Model file for the job. Use its own axes, mm. A direction names the side the tool comes from. Round coordinates to 2 decimals unless told otherwise and drop trailing zeros. Order: outer loops, then holes, each group sorted by start corner. A loop starts at its lowest first (then second) coordinate and runs counter-clockwise, first axis right, second up. Notation, with made-up numbers: (7, -31) - (66, -31) arc R18 ccw to (66, -23) - close; hole circle Ø2 at (-7, 54). An arc over 180 degrees is marked (long way). Put each result on its own line as item: value. Start each with the question number.
Item 1: Pin check, flat tip, straight feed: pin 1 Ø1 at (x, y) = (-16.5, 34) entering from +Z. Stop position of the tip, or through.
Item 2: Probe probe 1 along Y at (x, z) = (-40.5, 0.5); probe 2 along Y at (x, z) = (-11, 4); probe 3 along Y at (x, z) = (14, 2). List the from-to ranges inside material, lowest first.
Item 3: Which spindle directions (+Z, -Z, +X, -X, +Y, -Y) get a long thin tool onto all of the face, cutting with end or side? Do faces 1 (the face through (0, -32, 2)), 2 (the face through (2, -12.278, 2)). Say none if no direction does.
Item 4: Saw through at C-C on y = -10.5. List the corners of the cut face in (x, z), plus the area to 3 significant figures.
Item 5: Saw through at D-D on x = -43.5. List the corners of the cut face in (y, z).
Item 6: Mould opens along X. For faces 3 (the face through (1, -56.48, 2)), 4 (the face through (-38, -26.567, 2)) say: pulls with the +X half, pulls with the -X half, needs draft (parallel to the pull), parting line crosses it, or undercut.
Item 7: Saw through at A-A on x = 9. List the corners of the cut face in (y, z).
Item 8: Saw through at B-B on z = 2. List the corners of the cut face in (x, y), plus the area to 3 significant figures.
```python
from build123d import *

# Parameters (mm, degrees)
F1_DEPTH = 5
F2_DEPTH = 2


# Not quite as in the source:
# - a feature names something its author has since deleted; it is built from what else it names


with BuildPart() as f1:
    # F0 (on Top) → F1 (new body)
    with BuildSketch(Plane.XY):
        Polygon((-53.2781591106, 53.5204063327), (-53.2781591106, -56.4795936673), (-13.7344817631, -56.4795936673), (56.7218408894, -56.4795936673), (56.7218408894, 53.5204063327), align=None)
        Polygon((-49.0473898798, 29.4351325184), (-49.0473898798, 49.289637102), (52.4910716586, 49.289637102), (52.4910716586, 29.4351325184), (27.9224817305, -52.2488244365), (-13.7344817631, -52.2488244365), (-13.7344817631, -40.6398742527), (-26.4708319562, -40.6398742527), (-26.4708319562, -26.5670741801), (-49.0473898798, -26.5670741801), (-49.0473898798, 5.428542512), (-49.0473898798, 25.9305896417), (-26.4708319562, 25.9305896417), (13.9133328608, 25.9305896417), (13.9133328608, 5.428542512), (13.9133328608, -12.2777693511), (-9.5037125323, -12.2777693511), (-9.5037125323, 5.428542512), (-26.4708319562, 5.428542512), (-26.4708319562, -12.2777693511), (-13.7344817631, -12.2777693511), (-13.7344817631, -26.5670741801), (0, -26.5670741801), (0, -37.4845501322), (17.3598656954, -37.4845501322), (37.487713347, 29.4351325184), align=None, mode=Mode.SUBTRACT)
    extrude(amount=F1_DEPTH)

    # F0 (on Top) → F2 (join)
    with BuildSketch(Plane.XY):
        Polygon((-53.2781591106, 53.5204063327), (-53.2781591106, -56.4795936673), (-13.7344817631, -56.4795936673), (56.7218408894, -56.4795936673), (56.7218408894, 53.5204063327), align=None)
        Polygon((-49.0473898798, 29.4351325184), (-49.0473898798, 49.289637102), (52.4910716586, 49.289637102), (52.4910716586, 29.4351325184), (27.9224817305, -52.2488244365), (-13.7344817631, -52.2488244365), (-13.7344817631, -40.6398742527), (-26.4708319562, -40.6398742527), (-26.4708319562, -26.5670741801), (-49.0473898798, -26.5670741801), (-49.0473898798, 5.428542512), (-49.0473898798, 25.9305896417), (-26.4708319562, 25.9305896417), (13.9133328608, 25.9305896417), (13.9133328608, 5.428542512), (13.9133328608, -12.2777693511), (-9.5037125323, -12.2777693511), (-9.5037125323, 5.428542512), (-26.4708319562, 5.428542512), (-26.4708319562, -12.2777693511), (-13.7344817631, -12.2777693511), (-13.7344817631, -26.5670741801), (0, -26.5670741801), (0, -37.4845501322), (17.3598656954, -37.4845501322), (37.487713347, 29.4351325184), align=None, mode=Mode.SUBTRACT)
        Polygon((52.4910716586, 49.289637102), (-49.0473898798, 49.289637102), (-49.0473898798, 29.4351325184), (37.487713347, 29.4351325184), (17.3598656954, -37.4845501322), (0, -37.4845501322), (0, -26.5670741801), (-13.7344817631, -26.5670741801), (-13.7344817631, -12.2777693511), (-26.4708319562, -12.2777693511), (-26.4708319562, 5.428542512), (-9.5037125323, 5.428542512), (13.9133328608, 5.428542512), (13.9133328608, 25.9305896417), (-26.4708319562, 25.9305896417), (-49.0473898798, 25.9305896417), (-49.0473898798, 5.428542512), (-49.0473898798, -26.5670741801), (-26.4708319562, -26.5670741801), (-26.4708319562, -40.6398742527), (-13.7344817631, -40.6398742527), (-13.7344817631, -52.2488244365), (27.9224817305, -52.2488244365), (52.4910716586, 29.4351325184), align=None)
    extrude(amount=-F2_DEPTH)


solid = f1.part
```
Results found:
1. pin 1: stops at z = 0
2. probe 1: y = -56.48 to -26.57, 25.93 to 29.44, 49.29 to 53.52
2. probe 2: y = -56.48 to -52.25, -26.57 to 5.43, 25.93 to 29.44, 49.29 to 53.52
2. probe 3: y = -56.48 to -52.25, -37.48 to 29.44, 49.29 to 53.52
3. face 1: +Z
3. face 2: +Z, -Z
4. outline: (-53.28, -2) - (-9.5, -2) - (-9.5, 5) - (-26.47, 5) - (-26.47, 0) - (-49.05, 0) - (-49.05, 5) - (-53.28, 5) - close; (13.91, -2) - (56.72, -2) - (56.72, 5) - (40.48, 5) - (40.48, 0) - (25.48, 0) - (25.48, 5) - (13.91, 5) - close
4. area: 418 mm²
5. outline: (-56.48, -2) - (53.52, -2) - (53.52, 5) - (49.29, 5) - (49.29, 0) - (29.44, 0) - (29.44, 5) - (25.93, 5) - (25.93, 0) - (-26.57, 0) - (-26.57, 5) - (-56.48, 5) - close
6. face 3: needs draft
6. face 4: undercut
7. outline: (-56.48, -2) - (-12.28, -2) - (-12.28, 5) - (-37.48, 5) - (-37.48, 0) - (-52.25, 0) - (-52.25, 5) - (-56.48, 5) - close; (5.43, -2) - (53.52, -2) - (53.52, 5) - (49.29, 5) - (49.29, 0) - (29.44, 0) - (29.44, 5) - (25.93, 5) - (25.93, 0) - (5.43, 0) - close
8. outline: (-53.28, -56.48) - (56.72, -56.48) - (56.72, 53.52) - (-53.28, 53.52) - close; hole (-49.05, -26.57) - (-26.47, -26.57) - (-26.47, -40.64) - (-13.73, -40.64) - (-13.73, -52.25) - (27.92, -52.25) - (52.49, 29.44) - (52.49, 49.29) - (-49.05, 49.29) - (-49.05, 29.44) - (37.49, 29.44) - (17.36, -37.48) - (0, -37.48) - (0, -26.57) - (-13.73, -26.57) - (-13.73, -12.28) - (-26.47, -12.28) - (-26.47, 5.43) - (-9.5, 5.43) - (-9.5, -12.28) - (13.91, -12.28) - (13.91, 25.93) - (-49.05, 25.93) - close
8. area: 5,490 mm²
